Autodesk Fusion 360 part; units mm, degrees
sketch "Sketch1" plane through (0, 0, 0) normal (0, 0, 1) x (1, 0, 0)
  line L0 (-28, 37) -> (62, 37)
  line L1 (62, 37) -> (62, 18)
  line L2 (62, 18) -> (-28, 18)
  line L3 (-28, 18) -> (-28, 37)
  dimension "d1" = 90
  dimension "d2" = 19
extrude "Extrude1" add sketch "Sketch1" along normal blind 6
sketch "Sketch2" plane through (0, 0, 6) normal (0, 0, 1) x (-1, 0, 0)
  line L0 (28, -37) -> (28, -18)
  line L1 (28, -18) -> (-62, -18)
  line L2 (-62, -18) -> (-62, -37)
  line L3 (-62, -37) -> (28, -37)
ref_plane "WorkPlane1" through (17, 27.5, 6) normal (0, 0, 1) x (-1, 0, 0)
sketch "Sketch3" plane through (0, 0, 6) normal (0, 0, 1) x (1, 0, 0)
  line L0 (17, 37) -> (17, 18)
  circle A0 centre (-8, 27.5) radius 8.9
  circle A1 centre (42, 27.5) radius 8.9
  circle A2 centre (-8, 27.5) radius 3.65
  circle A3 centre (42, 27.5) radius 3.65
  dimension "d13" = 17.8
  dimension "d14" = 17.8
  dimension "d15" = 7.3
  dimension "d16" = 7.3
extrude "Extrude2" cut sketch "Sketch3" against normal blind 7 contours A2 | A3
extrude "Extrude3" cut sketch "Sketch3" against normal blind 3
sketch "Sketch7" plane through (0, 0, 0) normal (0, 0, -1) x (1, 0, 0)
  circle A0 centre (42, -27.5) radius 3.65
  circle A1 centre (-8, -27.5) radius 3.65
  line L0 (62, -18) -> (-28, -18)
  line L1 (-28, -18) -> (-28, -37)
  line L2 (-28, -37) -> (62, -37)
  line L3 (62, -37) -> (62, -18)
  line L4 (-28, -18) -> (62, -18)
  line L5 (62, -18) -> (62, -8)
  line L6 (62, -8) -> (-28, -8)
  line L7 (-28, -8) -> (-28, -18)
  dimension "d37" = 10
  dimension "d38" = 90
extrude "Extrude7" add sketch "Sketch7" against normal blind 6 contours L0 L4 L5 L6 L7
sketch "Sketch8" plane through (-28, 0, 0) normal (-1, 0, 0) x (0, -1, 0)
  line L0 (-37, 0) -> (-8, 0)
  line L1 (-8, 0) -> (-8, 6)
  line L2 (-8, 6) -> (-37, 6)
  line L3 (-37, 6) -> (-37, 0)
ref_plane "WorkPlane3" through (17, 22.5, 0) normal (0, 0, -1) x (-1, 0, 0)
sketch "Sketch9" plane through (0, 0, 0) normal (0, 0, -1) x (-1, 0, 0)
  line L0 (-62, 37) -> (28, 37)
  line L1 (28, 37) -> (28, 47)
  line L2 (28, 47) -> (-62, 47)
  line L3 (-62, 47) -> (-62, 37)
  dimension "d42" = 90
  dimension "d43" = 10
extrude "Extrude8" add sketch "Sketch9" against normal blind 6
ref_plane "WorkPlane4" through (17, 8, 3) normal (0, -1, 0) x (1, 0, 0)
sketch "Sketch10" plane through (0, 8, 0) normal (0, -1, 0) x (-1, 0, 0)
  line L0 (28, -6) -> (24, -6)
  line L1 (24, -6) -> (24, -57.5)
  line L2 (24, -57.5) -> (28, -57.5)
  line L3 (28, -57.5) -> (28, -6)
  dimension "d47" = 4
  dimension "d48" = 51.5
extrude "Extrude9" add sketch "Sketch10" against normal blind 39
sketch "Sketch11" plane through (0, 8, 0) normal (0, -1, 0) x (1, 0, 0)
  line L0 (-28, 0) -> (62, 0)
  line L1 (62, 0) -> (62, 6)
  line L2 (62, 6) -> (-24, 6)
  line L3 (-24, 6) -> (-24, 57.5)
  line L4 (-24, 57.5) -> (-28, 57.5)
  line L5 (-28, 57.5) -> (-28, 0)
  line L6 (-28, 57.5) -> (62, 57.5)
  line L7 (62, 57.5) -> (62, 53.5)
  line L8 (62, 53.5) -> (-28, 53.5)
  line L9 (-28, 53.5) -> (-28, 57.5)
  dimension "d51" = 90
  dimension "d52" = 4
extrude "Extrude10" add sketch "Sketch11" against normal blind 39 contours L3 L6 L7 L8
sketch "Sketch12" plane through (0, 8, 0) normal (0, -1, 0) x (1, 0, 0)
  line L0 (-28, 0) -> (62, 0)
  line L1 (62, 0) -> (62, 6)
  line L2 (62, 6) -> (-24, 6)
  line L3 (-24, 6) -> (-24, 53.5)
  line L4 (-24, 53.5) -> (62, 53.5)
  line L5 (62, 53.5) -> (62, 57.5)
  line L6 (62, 57.5) -> (-28, 57.5)
  line L7 (-28, 57.5) -> (-28, 0)
  circle A0 centre (-24, 6) radius 22.25
  line L8 (-24, 28.25) -> (62, 28.25)
  line L9 (62, 28.25) -> (62, 31.25)
  line L10 (62, 31.25) -> (-24, 31.25)
  line L11 (-24, 31.25) -> (-24, 28.25)
  dimension "d55" = 44.5
  dimension "d56" = 86
  dimension "d57" = 3
extrude "Extrude11" add sketch "Sketch12" against normal blind 39 contours L3 L8 L9 L10 L11
fillet "Fillet3" radius 2 1 edges at (-28, 27.5, 57.5)
fillet "Fillet4" radius 2 1 edges at (-28, 27.5, 0)
fillet "Fillet5" radius 2 2 edges at (-24, 27.5, 53.5) (-24, 27.5, 28.25)
fillet "Fillet6" radius 2 2 edges at (-24, 27.5, 31.25) (-24, 27.5, 6)
fillet "Fillet7" radius 1 2 edges at (62, 27.5, 31.25) (62, 27.5, 28.25)
fillet "Fillet8" radius 2 4 edges at (62, 27.5, 57.5) (62, 27.5, 53.5) (62, 27.5, 6) (62, 27.5, 0)
Input: part model. Units: mm. Frame: model coordinates. A direction names the side the tool comes from. Coordinates: 2 decimals unless noted, no trailing zeros. Loops run counter-clockwise (first coordinate to the right, second up) from the corner with the lowest first, then second, coordinate; pieces in that order, holes last.
Q1. Section B-B, the plane x = 13. Return the cut outline in (y, z), and give its area (3 significant figures).
Results are:
outline: (8, 0) - (47, 0) - (47, 6) - (8, 6) - close; (8, 28.25) - (47, 28.25) - (47, 31.25) - (8, 31.25) - close; (8, 53.5) - (47, 53.5) - (47, 57.5) - (8, 57.5) - close
area: 507 mm2
Q2. Section A-A, the plane x = 42. Return the cut outline in (y, z), and give its area (3 significant figures).
Results are:
outline: (8, 0) - (23.85, 0) - (23.85, 3) - (18.6, 3) - (18.6, 6) - (8, 6) - close; (8, 28.25) - (47, 28.25) - (47, 31.25) - (8, 31.25) - close; (8, 53.5) - (47, 53.5) - (47, 57.5) - (8, 57.5) - close; (31.15, 0) - (47, 0) - (47, 6) - (36.4, 6) - (36.4, 3) - (31.15, 3) - close
area: 432 mm2
Q3. Line query: line 1 along Z through (x, y) = (15, 27); line 2 along Z through (x, y) = (-16, 30.5); line 3 along Y through (x, z) = (-8, 1.7). Output: solid intervals per line, ascending.
Results are:
line 1: z = 0 to 6, 28.25 to 31.25, 53.5 to 57.5
line 2: z = 0 to 3, 28.25 to 31.25, 53.5 to 57.5
line 3: y = 8 to 23.85, 31.15 to 47
Q4. Set-up query: faces 5 (the flat face through (20, 28, 6)), 6 (the cylindrical face through (-3.9, 19.6, 4.5)), 7 (the cylindrical face through (39.103, 25.279, 1.521)). Return all of +Z, -Z, +X, -X, +Y, -Y with unobstructed straight access to the full face (end or side cutting, diameter ignored); none if empty.
Results are:
face 5: +X, +Y, -Y
face 6: none
face 7: -Z
Q5. Contact query for a flat-ended pin moving along its axis: pin 1 (5.5 mm diameter, centred on y = 20, z = 38, fed in from +X). Output: stop coordinate, or through.
Results are:
pin 1: stops at x = -24
Q6. Mould query, pull axis X, two halves, no side actions, for faces 1 (the flat face through (46, 28, 3)), 2 (the cylindrical face through (61.4, 27.77, 56.93)), 3 (the flat face through (13, 8, 29)), 4 (the cylindrical face through (-8.791, 23.937, 1.521)). Classes: +X half, -X half, draft (parallel to the pull), parting line (faces both ways), or undercut.
Results are:
face 1: undercut
face 2: +X half
face 3: draft
face 4: undercut
Q7. Section C-C, the plane y = 27.5. Give the number of separate pieces and of enclosed holes in the cut face, and give its area (3 significant figures).
Results are:
separate pieces: 3
enclosed holes: 0
area: 1,200 mm2
